Design review of the part built by this model. Coordinates are the model's own, in mm. Give positions to 0.01 mm unless a question says otherwise; leave off trailing zeros. Loops run counter-clockwise (first coordinate to the right, second up) from the corner with the lowest first, then second, coordinate; pieces in that order, holes last. Notation, with made-up numbers: (-24.5, 22) -> (-11.5, 22) arc R14 ccw to (-11.5, 47) -> close; hole circle Ø5 at (-2.5, 61.5). An arc over 180 degrees is marked (long way). Use CSV: the item, a comma, the result in double quotes. Start each with the question number.
Item 1: We need section D-D (y = -4.75). State the section outline as (x, z) points.
Item 2: The part is to be moulded in two halves that separate along X. For faces 1 (the face through (1.802, -0.084, 5.723)), 2 (the face through (11.94, 0.07, 7.03)), 3 (the face through (-12.056, 0.075, 6.831)), 4 (the face through (5, 6, 5)), say which applies: +X half, -X half, draft (parallel to the pull), parting line (faces both ways), or undercut.
Item 3: We need section C-C (y = 2). State the section outline as (x, z) points, plus the area to 3 significant figures.
Item 4: We need section A-A (y = 0.25). State the section outline as (x, z) points, plus the area to 3 significant figures.
Item 5: Wall thickness on line 1 along Z through (x, y) = (-4, 2.75); line 2 along X through (y, z) = (-5.25, -5); line 3 along Z through (x, y) = (-3.5, 3): over which ranges is each line inside the solid? List them lowest first. Write a range as from..to.
Item 6: We need section B-B (x = 0). State the section outline as (y, z) points, plus the area to 3 significant figures.
Item 7: Clearance check with flat-ended pins moving along their axes: pin 1 (4 mm diameter, centred on y = -1, z = 6.5, fed in from -X); pin 2 (8 mm diameter, centred on x = -11, z = 9, fed in from -Y); pin 3 (3 mm diameter, centred on y = -2.5, z = -9.5, fed in from -X); pin 4 (3 mm diameter, centred on y = -3.5, z = -10, fed in from +X). State where each tip first meets the part, or that it passes through.
from build123d import *

# Parameters (mm, degrees)
SKETCH1_R           = 6
BOSS_EXTRUDE1_DEPTH = 6


with BuildPart() as part:
    # Sketch1 → Boss-Extrude1 (new, symmetric)
    with BuildSketch(Plane(origin=(0, 0, 0), x_dir=(1, 0, 0), z_dir=(0, 1, 0))):
        Polygon((16, 0), (8, 13.856406461), (-8, 13.856406461), (-16, 0), (-8, -13.856406461), (8, -13.856406461), align=None)
        with Locations(Location((0, 0, 0), (0, 0, 270))):
            Circle(SKETCH1_R, mode=Mode.SUBTRACT)
    extrude(amount=BOSS_EXTRUDE1_DEPTH, both=True)

    # Sketch2 → Cut-Revolve2 (revolve, cut)
    with BuildSketch(Plane.XY, mode=Mode.PRIVATE) as cut_revolve2_sk:
        with BuildLine():
            Line((11.5, 6), (16, 6))
            Line((16, 6), (16, 1.5))
            ThreePointArc((16, 1.5), (14.681980515, 4.681980515), (11.5, 6))
        make_face()
        with BuildLine():
            Line((11.5, -6), (16, -6))
            Line((16, -6), (16, -1.5))
            ThreePointArc((16, -1.5), (14.681980515, -4.681980515), (11.5, -6))
        make_face()
    revolve(cut_revolve2_sk.sketch.rotate(Axis((0, 9.943732914, 0), (0, -1, 0)), 90), axis=Axis((0, 9.943732914, 0), (0, -1, 0)), mode=Mode.SUBTRACT)


solid = part.part
Results found:
1,outline,"(-14.32, -2.91) -> (-9.68, -10.95) arc R14.61 ccw to (-4.64, -13.86) -> (4.64, -13.86) arc R14.61 ccw to (9.68, -10.95) -> (14.32, -2.91) arc R14.61 ccw to (14.32, 2.91) -> (9.68, 10.95) arc R14.61 ccw to (4.64, 13.86) -> (-4.64, 13.86) arc R14.61 ccw to (-9.68, 10.95) -> (-14.32, 2.91) arc R14.61 ccw to start; hole circle Ø12 at (0, 0)"
2,face 1,"undercut"
2,face 2,"+X half"
2,face 3,"-X half"
2,face 4,"draft"
3,outline,"(-15.97, -0.05) -> (-8.03, -13.81) arc R15.97 ccw to (-7.94, -13.86) -> (7.94, -13.86) arc R15.97 ccw to (8.03, -13.81) -> (15.97, -0.05) arc R15.97 ccw to (15.97, 0.05) -> (8.03, 13.81) arc R15.97 ccw to (7.94, 13.86) -> (-7.94, 13.86) arc R15.97 ccw to (-8.03, 13.81) -> (-15.97, 0.05) arc R15.97 ccw to start; hole circle Ø12 at (0, 0)"
3,area,"552 mm²"
4,outline,"(-16, 0) -> (-8, -13.86) -> (8, -13.86) -> (16, 0) -> (8, 13.86) -> (-8, 13.86) -> close; hole circle Ø12 at (0, 0)"
4,area,"552 mm²"
5,line 1,"-13.86..-4.47, 4.47..13.86"
5,line 2,"-13.06..-3.32, 3.32..13.06"
5,line 3,"-13.86..-4.87, 4.87..13.86"
6,outline,"(-6, -11.5) arc R4.5 ccw to (-5.33, -13.86) -> (5.33, -13.86) arc R4.5 ccw to (6, -11.5) -> (6, -6) -> (-6, -6) -> close; (-6, 6) -> (6, 6) -> (6, 11.5) arc R4.5 ccw to (5.33, 13.86) -> (-5.33, 13.86) arc R4.5 ccw to (-6, 11.5) -> close"
6,area,"187 mm²"
7,pin 1,"x = -13.4"
7,pin 2,"y = -6"
7,pin 3,"x = -11.38"
7,pin 4,"x = 11.09"
